Input: dimensioned drawing with shaded views. Units: mm. Origin: part minimum x, y, z. A direction names the side the tool comes from. Coordinates: 2 decimals unless noted, no trailing zeros. Loops run counter-clockwise (first coordinate to the right, second up) from the corner with the lowest first, then second, coordinate; pieces in that order, holes last.
Item 1: Pull-direction query (Z, two-part tool) for the marked faces 5, 6 and 7; classes: +Z half, -Z half, draft (parallel to the pull), parting line (faces both ways), or undercut.
Item 2: Section query A-A, the plane x = 6.5. Return the cut outline in (y, z) (1 decimal).
Item 3: Section query B-B, the plane z = 12.7. Return the cut outline in (x, y).
Item 4: Section query D-D, the plane x = 12.25. Return the cut outline in (y, z) (1 decimal).
Item 5: Pin query (flat end, axial travel): pin 1 Ø4.5 at (x, y) = (21.5, 2.5) entering from -Z; pin 2 Ø3 at (x, y) = (21.5, 3) entering from +Z; pin 3 Ø1.5 at (x, y) = (20.5, 8) entering from +Z (1 decimal). Return the tip coordinate at first contact, or that it passes through.
Item 6: Section query C-C, the plane y = 4.75. Return the cut outline in (x, z) (1 decimal).
Item 7: Reachability of the marked faces 1, 2, 3 and 4 from +Z, -Z, +X, -X, +Y, -Y: full face, straight path, thin tool, end or side. Return the list, or none.
Item 8: Line query: probe 1 along Y at (x, z) = (9.5, 22.5); probe 2 along X at (y, z) = (3.25, 20.75) (1 decimal); probe 3 along Z at (x, y) = (16, 2) (1 decimal). Output: solid intervals per line, ascending.
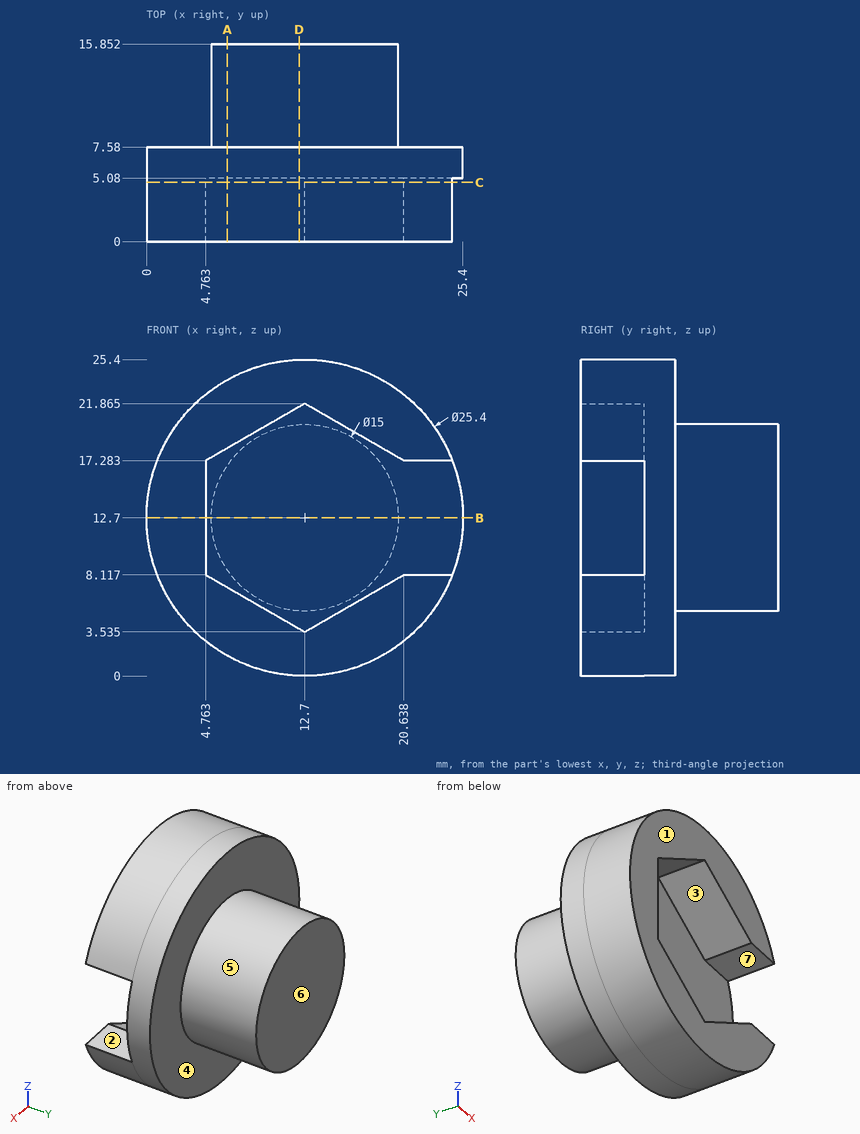
Verdict:
1. face 5: parting line
1. face 6: draft
1. face 7: undercut
2. outline: (0, 1.6) - (7.6, 1.6) - (7.6, 8.5) - (15.9, 8.5) - (15.9, 16.9) - (7.6, 16.9) - (7.6, 23.8) - (0, 23.8) - (0, 18.3) - (5.1, 18.3) - (5.1, 7.1) - (0, 7.1) - close
3. outline: (0, 0) - (4.76, 0) - (4.76, 5.08) - (25.4, 5.08) - (25.4, 7.58) - (20.2, 7.58) - (20.2, 15.85) - (5.2, 15.85) - (5.2, 7.58) - (0, 7.58) - close
4. outline: (0, 0) - (7.6, 0) - (7.6, 5.2) - (15.9, 5.2) - (15.9, 20.2) - (7.6, 20.2) - (7.6, 25.4) - (0, 25.4) - (0, 21.6) - (5.1, 21.6) - (5.1, 3.8) - (0, 3.8) - close
5. pin 1: stops at z = 1.82
5. pin 2: stops at z = 23.09
5. pin 3: stops at z = 23.2
6. outline: (4.8, 8.1) - (4.8, 17.3) - (12.7, 21.9) - (20.6, 17.3) - (24.5, 17.3) arc R12.7 ccw (long way) to (24.5, 8.1) - (20.6, 8.1) - (12.7, 3.5) - close
7. face 1: +Z, -Z, +X, -X, -Y
7. face 2: +X, -Y
7. face 3: -Y
7. face 4: +Y
8. probe 1: y = 0 to 7.58
8. probe 2: x = 2.9 to 10.8, 14.6 to 22.5
8. probe 3: z = 0.4 to 5.4, 20 to 25
